```python
from build123d import *

# Parameters (mm, degrees)
SKETCH1_W           = 210
SKETCH1_H           = 220
BOSS_EXTRUDE1_DEPTH = 1555
SKETCH2_W           = 937
SKETCH2_H           = 163
CUT_EXTRUDE1_DEPTH  = 7
SKETCH4_W           = 163
SKETCH4_H           = 937
CUT_EXTRUDE2_DEPTH  = 7
SKETCH5_W           = 270
SKETCH5_H           = 270
BOSS_EXTRUDE2_DEPTH = 140
CHAMFER1_SIZE       = 25
FILLET1_R           = 20
BOSS_EXTRUDE3_DEPTH = 20


with BuildPart() as part:
    # Sketch1 → Boss-Extrude1 (new body)
    with BuildSketch(Plane.XY):
        Rectangle(SKETCH1_W, SKETCH1_H)
    extrude(amount=BOSS_EXTRUDE1_DEPTH)

    # Sketch2 → Cut-Extrude1 (cut)
    with BuildSketch(Plane.ZY.offset(105)):
        with Locations((946.5, 0)):
            Rectangle(SKETCH2_W, SKETCH2_H)
    cut_extrude1 = extrude(amount=-CUT_EXTRUDE1_DEPTH, mode=Mode.SUBTRACT)

    # Mirror2: Cut-Extrude1 across plane
    add(cut_extrude1.mirror(Plane(origin=(0, 0, 0), x_dir=(0, 0, 1), z_dir=(1, 0, 0))), mode=Mode.SUBTRACT)

    # Sketch4 → Cut-Extrude2 (cut)
    with BuildSketch(Plane(origin=(0, 110, 0), x_dir=(1, 0, 0), z_dir=(0, 1, 0))):
        with Locations((0, -946.5)):
            Rectangle(SKETCH4_W, SKETCH4_H)
    cut_extrude2 = extrude(amount=-CUT_EXTRUDE2_DEPTH, mode=Mode.SUBTRACT)

    # Mirror3: Cut-Extrude2 across plane
    add(cut_extrude2.mirror(Plane.ZX), mode=Mode.SUBTRACT)

    # Sketch5 → Boss-Extrude2 (add)
    with BuildSketch(Plane.XY.offset(1555)):
        Rectangle(SKETCH5_W, SKETCH5_H)
    extrude(amount=-BOSS_EXTRUDE2_DEPTH)

    # Chamfer1
    chamfer1_edges = [part.edges().sort_by_distance(p)[0] for p in [
        (135, 0, 1555),
        (0, 135, 1555),
        (-135, 0, 1555),
        (0, -135, 1555),
    ]]
    chamfer(chamfer1_edges, length=CHAMFER1_SIZE)

    # Fillet1
    fillet1_edges = [part.edges().sort_by_distance(p)[0] for p in [
        (122.5, 122.5, 1542.5),
        (122.5, -122.5, 1542.5),
        (-122.5, 122.5, 1542.5),
        (-122.5, -122.5, 1542.5),
    ]]
    fillet(fillet1_edges, radius=FILLET1_R)

    # Sketch6 → Boss-Extrude3 (add)
    with BuildSketch(Plane(origin=(0, 0, 0), x_dir=(-1, 0, 0), z_dir=(0, 0, -1))):
        Polygon((-20, 135), (20, 135), (20, 20), (135, 20), (135, -20), (20, -20), (20, -135), (-20, -135), (-20, -20), (-135, -20), (-135, 20), (-20, 20), align=None)
    extrude(amount=-BOSS_EXTRUDE3_DEPTH)


solid = part.part
```
Input: part model. Units: mm. Frame: model coordinates. A direction names the side the tool comes from. Coordinates: 2 decimals unless noted, no trailing zeros. Write each loop counter-clockwise with the first axis right and the second up, starting at its lowest first coordinate (ties: lowest second). Pieces come first, ordered by that corner, then holes. Notation, with made-up numbers: (-6.75, 4.5) - (35.25, 4.5) arc R36 ccw to (35.25, 40.5) - close; hole circle Ø1 at (11, 29.5). An arc over 180 degrees is marked (long way). Put each result on its own line as item: value. Start each with the question number.
1) Reachability of faces 5 (the face through (118, 2, 1415)), 6 (the face through (-120, 0, 20)), 7 (the face through (98, 1, 940)) from +Z, -Z, +X, -X, +Y, -Y: full face, straight path, thin tool, end or side. Return the list, or none.
2) Cut plane C-C (x = -44). Return the cut outline in (y, z).
3) Cut plane A-A (z = 1034). Return the cut outline in (x, y), plus the area to 3 significant figures.
4) Cut plane D-D (z = 287). Return the cut outline in (x, y).
5) Mould query, pull axis Y, two halves, no side actions, for faces 1 (the face through (105, -2, 383)), 2 (the face through (-119.398, 119.191, 1541.916)), 3 (the face through (-98, 1, 940)), 4 (the face through (119.624, -119.832, 1541.482)). Classes: pulls with the +Y half, pulls with the -Y half, needs draft (parallel to the pull), parting line crosses it, or undercut.
6) Contact query for flat-ended pins moving along their axis: pin 1 (12 mm diameter, centred on y = 35, z = 1239.5, fed in from +X); pin 2 (10 mm diameter, centred on y = -66, z = 305.5, fed in from +X); pin 3 (22 mm diameter, centred on y = -128.5, z = 11, fed in from -X). Output: stop coordinate, or through.
7) Cut plane B-B (y = -42). Return the cut outline in (x, z), plus the area to 3 significant figures.
8) Ray query, L1, parallel to Y at x = -101.5, z = 649; L2, parallel to Z at x = -100.5, y = -43; L3, parallel to Y at x = 61, z = 377. Return the intervals inside material, ascending.
Resolved:
1. face 5: none
1. face 6: -X, +Y, -Y
1. face 7: +X
2. outline: (-135, 1415) - (-103, 1415) - (-103, 478) - (-110, 478) - (-110, 0) - (110, 0) - (110, 478) - (103, 478) - (103, 1415) - (135, 1415) - (135, 1530) - (110, 1555) - (-110, 1555) - (-135, 1530) - close
3. outline: (-105, -110) - (-81.5, -110) - (-81.5, -103) - (81.5, -103) - (81.5, -110) - (105, -110) - (105, -81.5) - (98, -81.5) - (98, 81.5) - (105, 81.5) - (105, 110) - (81.5, 110) - (81.5, 103) - (-81.5, 103) - (-81.5, 110) - (-105, 110) - (-105, 81.5) - (-98, 81.5) - (-98, -81.5) - (-105, -81.5) - close
3. area: 41,600 mm2
4. outline: (-105, -110) - (105, -110) - (105, 110) - (-105, 110) - close
5. face 1: needs draft
5. face 2: pulls with the +Y half
5. face 3: undercut
5. face 4: pulls with the -Y half
6. pin 1: stops at x = 98
6. pin 2: stops at x = 105
6. pin 3: stops at x = -20
7. outline: (-135, 1415) - (-98, 1415) - (-98, 478) - (-105, 478) - (-105, 0) - (105, 0) - (105, 478) - (98, 478) - (98, 1415) - (135, 1415) - (135, 1530) - (110, 1555) - (-110, 1555) - (-135, 1530) - close
7. area: 321,000 mm2
8. L1: y = -110 to -81.5, 81.5 to 110
8. L2: z = 0 to 478, 1415 to 1555
8. L3: y = -110 to 110
